```python
from build123d import *

# Parameters (mm, degrees)
F0_W      = 250.311822
F0_H      = 106.41057
F1_DEPTH  = 57.15
F2_W      = 246.1734
F2_H      = 107.510934
F3_DEPTH  = 44.958
F4_W      = 78.823588
F4_H      = 42.86033
F4_W_2    = 84.242716
F5_DEPTH  = 207.518
F6_W      = 47.32091
F6_H      = 5.413929
F7_DEPTH  = 56.388
F9_DEPTH  = 37.084
F10_R     = 7.910412
F11_R     = 6.211921
F12_W     = 47.843273
F12_H     = 89.287125
F13_DEPTH = 78.74


with BuildPart() as f1:
    # F0 (on Front) → F1 (new body, symmetric)
    with BuildSketch(Plane.XZ):
        Rectangle(F0_W, F0_H)
    extrude(amount=F1_DEPTH, both=True)

    # F2 (on Top) → F3 (cut, symmetric)
    with BuildSketch(Plane.XY):
        Rectangle(F2_W, F2_H)
    extrude(amount=F3_DEPTH, both=True, mode=Mode.SUBTRACT)

    # F4 (on Front) → F5 (cut, symmetric)
    with BuildSketch(Plane.XZ):
        with Locations((-73.158145, 21.79965)):
            Rectangle(F4_W, F4_H)
        with Locations((76.606676, 21.79965)):
            Rectangle(F4_W_2, F4_H)
    extrude(amount=F5_DEPTH, both=True, mode=Mode.SUBTRACT)

    # F6 (on Front) → F7 (join, symmetric)
    with BuildSketch(Plane.XZ):
        with Locations((-147.265818, 20.498943)):
            Rectangle(F6_W, F6_H)
        Polygon((-170.926273, 17.791979), (-170.926273, 23.205908), (-182.093537, 42.867189), (-184.512094, 41.480076), align=None)
    extrude(amount=F7_DEPTH, both=True)

    # F8 (on Front) → F9 (join, symmetric)
    with BuildSketch(Plane.XZ):
        with BuildLine():
            Line((-121.890865, 20.348705), (-171.379492, 20.264825))
            Line((-171.379492, 20.264825), (-140.906081, 9.599128))
            ThreePointArc((-140.906081, 9.599128), (-126.654572, -2.899753), (-125.059903, -21.788495))
            Line((-125.059903, -21.788495), (-117.50719, -19.347493))
            Line((-117.50719, -19.347493), (-121.890865, 20.348705))
        make_face()
    extrude(amount=F9_DEPTH, both=True)

    # F10
    f10_edges = [f1.edges().sort_by_distance(p)[0] for p in [
        (-144.735065, -37.084, 17.791979),
        (-125.155911, -37.084, 5.621087),
        (-125.155911, 37.084, 5.621087),
        (-144.735065, 37.084, 17.791979),
    ]]
    fillet(f10_edges, radius=F10_R)

    # F11
    f11_edges = [f1.edges().sort_by_distance(p)[0] for p in [
        (-125.155911, 41.039206, -6.549804),
        (-125.155911, 0, -6.549804),
        (-125.155911, -41.039206, -6.549804),
    ]]
    fillet(f11_edges, radius=F11_R)

    # F12 (on Front) → F13 (cut, symmetric)
    with BuildSketch(Plane.XZ):
        with Locations((0.642964, -1.218934)):
            Rectangle(F12_W, F12_H)
    extrude(amount=F13_DEPTH, both=True, mode=Mode.SUBTRACT)


solid = f1.part
```
Input: part model. Units: mm. Frame: model coordinates. A direction names the side the tool comes from. Coordinates: 2 decimals unless noted, no trailing zeros. Order: outer loops, then holes, each group sorted by start corner. A loop starts at its lowest first (then second) coordinate and runs counter-clockwise, first axis right, second up. Notation, with made-up numbers: (13.25, -33) - (42.25, -33) arc R38 cw to (42.25, 5) - close; hole circle Ø6 at (41, 86.25). An arc over 180 degrees is marked (long way). Put each result on its own line as item: value.
1. Cut plane C-C on y = 49.5. Return the cut outline in (x, z).
Report:
outline: (-184.51, 41.48) - (-170.93, 17.79) - (-125.16, 17.79) - (-125.16, -53.21) - (125.16, -53.21) - (125.16, 53.21) - (-125.16, 53.21) - (-125.16, 23.21) - (-170.93, 23.21) - (-182.09, 42.87) - close; hole (-123.09, -44.96) - (-23.28, -44.96) - (-23.28, -45.86) - (24.56, -45.86) - (24.56, -44.96) - (123.09, -44.96) - (123.09, 44.96) - (-123.09, 44.96) - close
2. Cut plane B-B on x = -63.5. Return the cut outline in (y, z).
Report:
outline: (-57.15, -53.21) - (57.15, -53.21) - (57.15, 0.37) - (53.76, 0.37) - (53.76, -44.96) - (-53.76, -44.96) - (-53.76, 0.37) - (-57.15, 0.37) - close; (-57.15, 43.23) - (-53.76, 43.23) - (-53.76, 44.96) - (53.76, 44.96) - (53.76, 43.23) - (57.15, 43.23) - (57.15, 53.21) - (-57.15, 53.21) - close
3. Line query: line 1 along Z through (x, y) = (-5, -2.5); line 2 along Y through (x, z) = (-105, -19.5); line 3 along Z through (x, y) = (32.5, -16). Output: solid intervals per line, ascending.
Report:
line 1: z = -53.21 to -45.86, 44.96 to 53.21
line 2: y = -57.15 to -53.76, 53.76 to 57.15
line 3: z = -53.21 to -44.96, 44.96 to 53.21
4. Reachability of faces 4 (the face through (-155, -56.388, 23)), 5 (the face through (-121, -37.084, -5)), 6 (the face through (-140.66, 40.53, 16.41)) from +Z, -Z, +X, -X, +Y, -Y: full face, straight path, thin tool, end or side. Return the list, or none.
Report:
face 4: +Z, -Z, -X, -Y
face 5: none
face 6: -Z, -X, +Y
5. Cut plane D-D on x = 27.5. Return the cut outline in (y, z).
Report:
outline: (-57.15, -53.21) - (57.15, -53.21) - (57.15, 53.21) - (-57.15, 53.21) - close; hole (-53.76, -44.96) - (53.76, -44.96) - (53.76, 44.96) - (-53.76, 44.96) - close
6. Contact query for flat-ended pins moving along their axis: pin 1 Ø1 at (y, z) = (-55, 26.5) entering from -X; pin 2 Ø2.5 at (x, z) = (-138, 8) entering from +Y; pin 3 Ø2.5 at (x, z) = (-137, 6.5) entering from -Y. Output: stop coordinate, or through.
Report:
pin 1: stops at x = -176.21
pin 2: stops at y = 37.08
pin 3: stops at y = -37.08
7. Draft query along Y for faces 1 (the face through (-29, 53.755, -9)), 2 (the face through (-152.77, -0.63, 13.75)), 3 (the face through (-140.66, -40.53, 16.41)). Return one class per face: pulls with the +Y half, pulls with the -Y half, needs draft (parallel to the pull), parting line crosses it, or undercut.
Report:
face 1: undercut
face 2: needs draft
face 3: pulls with the -Y half
8. Cut plane A-A on z = -31. Return the cut outline in (x, y).
Report:
outline: (-125.16, -57.15) - (-23.28, -57.15) - (-23.28, -53.76) - (-123.09, -53.76) - (-123.09, 53.76) - (-23.28, 53.76) - (-23.28, 57.15) - (-125.16, 57.15) - close; (24.56, -57.15) - (125.16, -57.15) - (125.16, 57.15) - (24.56, 57.15) - (24.56, 53.76) - (123.09, 53.76) - (123.09, -53.76) - (24.56, -53.76) - close
